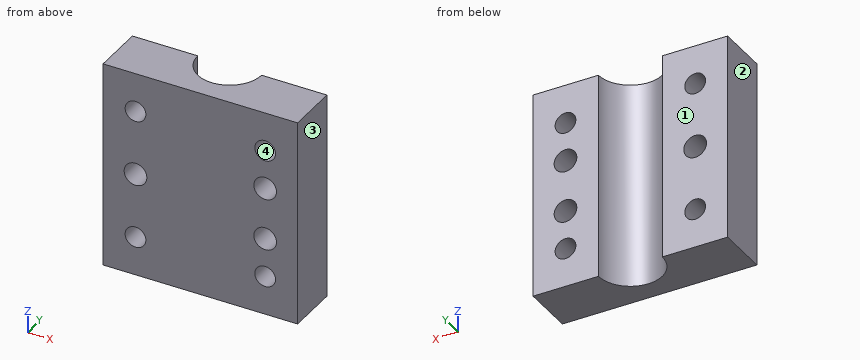
from build123d import *

# Parameters (mm, degrees)
SKETCH063_W     = 30
SKETCH063_H     = 32
SKETCH063_R     = 1.75
PAD039_DEPTH    = 8
SKETCH064_R     = 4.925
POCKET025_DEPTH = 38
SKETCH065_R     = 1.6
POCKET026_DEPTH = 10


with BuildPart() as part:
    # Sketch063 → Pad039 (new body)
    with BuildSketch(Plane.XZ):
        Rectangle(SKETCH063_W, SKETCH063_H)
        with Locations((-10, 0)):
            Circle(SKETCH063_R, mode=Mode.SUBTRACT)
        with Locations((10, 4)):
            Circle(SKETCH063_R, mode=Mode.SUBTRACT)
        with Locations((10, -4)):
            Circle(SKETCH063_R, mode=Mode.SUBTRACT)
    extrude(amount=PAD039_DEPTH)

    # Sketch064 (on Face3 of Pad039) → Pocket025 (cut)
    with BuildSketch(Plane(origin=(0, 0, -16), x_dir=(1, 0, 0), z_dir=(0, 0, -1))):
        Circle(SKETCH064_R)
    extrude(amount=-POCKET025_DEPTH, mode=Mode.SUBTRACT)

    # Sketch065 (on Face2 of Pocket025) → Pocket026 (cut)
    with BuildSketch(Plane(origin=(0, 0, 0), x_dir=(1, 0, 0), z_dir=(0, 1, 0))):
        with Locations((26.925, 5)):
            Circle(SKETCH065_R)
        with Locations((-10, 10)):
            Circle(SKETCH065_R)
        with Locations((10, 10)):
            Circle(SKETCH065_R)
        with Locations((10, -10)):
            Circle(SKETCH065_R)
        with Locations((-10, -10)):
            Circle(SKETCH065_R)
    extrude(amount=-POCKET026_DEPTH, mode=Mode.SUBTRACT)


with BuildPart() as part_1:
    # Body011 placement: moved
    add(part.part.moved(Location((-1.1, -53.7, 39.5))))


solid = part_1.part
Build history of the part. All positions in model axes, mm. Face numbers are marked on the shaded views. Give positions to 0.01 mm unless a question says otherwise; leave off trailing zeros. Order: outer loops, then holes, each group sorted by start corner. A loop starts at its lowest first (then second) coordinate and runs counter-clockwise, first axis right, second up. Notation, with made-up numbers: M 56.5,22.25 L 97.5,22.25 A11 ccw 97.5,30.25 Z; hole C 56.25,58.5 d11. An arc over 180 degrees is marked long. Put each result on its own line as item: value.
Item 1: Slice it at A-A, the plane z = 35.5. Write the cut outline in (x, y) (3 decimals).
From the geometry:
outline: M -16.1,-61.7 L 7.15,-61.7 L 7.15,-53.7 L 3.825,-53.7 A4.925 cw -6.025,-53.7 L -16.1,-53.7 Z; M 10.65,-61.7 L 13.9,-61.7 L 13.9,-53.7 L 10.65,-53.7 Z
Item 2: Slice it at C-C, the plane x = -11.1. Write the cut outline in (y, z), plus the area to 3 significant figures.
From the geometry:
outline: M -61.7,23.5 L -53.7,23.5 L -53.7,27.9 L -61.7,27.9 Z; M -61.7,31.1 L -53.7,31.1 L -53.7,37.75 L -61.7,37.75 Z; M -61.7,41.25 L -53.7,41.25 L -53.7,47.9 L -61.7,47.9 Z; M -61.7,51.1 L -53.7,51.1 L -53.7,55.5 L -61.7,55.5 Z
area: 177 mm2
Item 3: Slice it at B-B, the plane z = 29.5. Write the cut outline in (x, y) (3 decimals), plus the area to 3 significant figures.
From the geometry:
outline: M -16.1,-61.7 L -12.7,-61.7 L -12.7,-53.7 L -16.1,-53.7 Z; M -9.5,-61.7 L 7.3,-61.7 L 7.3,-53.7 L 3.825,-53.7 A4.925 cw -6.025,-53.7 L -9.5,-53.7 Z; M 10.5,-61.7 L 13.9,-61.7 L 13.9,-53.7 L 10.5,-53.7 Z
area: 151 mm2
Item 4: Probe line 1 (Z direction, x = 8.9, y = -56.5); line 2 (X direction, y = -55.25, z = 49); line 3 (Z direction, x = -10.75, y = -59). List the from-to ranges inside material, lowest first. Write a range as [from, to].
From the geometry:
line 1: z = [23.5, 27.9], [31.1, 33.75], [37.25, 41.75], [45.25, 47.9], [51.1, 55.5]
line 2: x = [-16.1, -12.62], [-9.58, -5.77], [3.57, 7.38], [10.42, 13.9]
line 3: z = [23.5, 27.94], [31.06, 37.79], [41.21, 47.94], [51.06, 55.5]
Item 5: Slice it at D-D, the plane y = -55.5. Give the number of separate pieces and of enclosed holes in the cut face, plus the area to 3 significant figures.
From the geometry:
separate pieces: 2
enclosed holes: 7
area: 606 mm2
Item 6: Two-plate mould, pull along X, no slides. Class the marked faces 1, 2, 3 and 4: +X half, -X half, draft (parallel to the pull), parting line (faces both ways), or undercut.
From the geometry:
face 1: draft
face 2: -X half
face 3: +X half
face 4: undercut
Item 7: Flat gauge pin, fed straight in: pin 1 Ø4.5 at (x, z) = (8.9, 35.5) entering from -Y. Where does the tip first touch, or does it go through?
From the geometry:
pin 1: stops at y = -61.7
